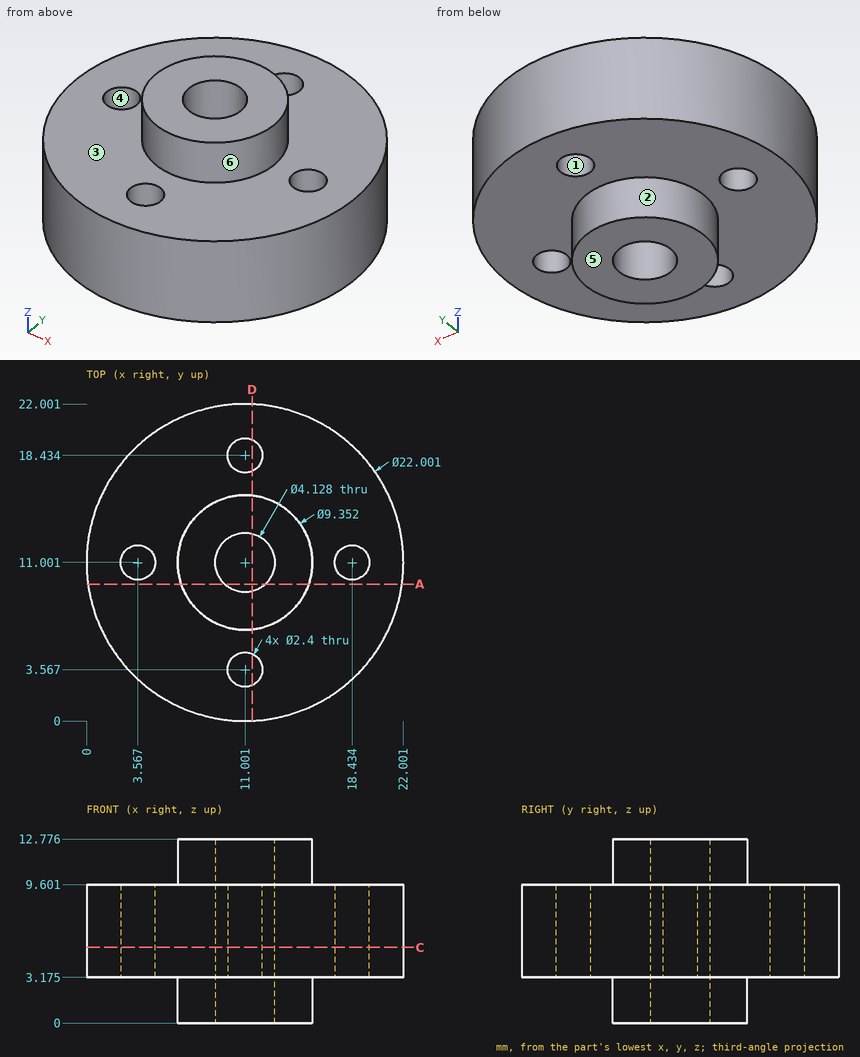
Geometry: see drawing. Coordinates: mm, zero at the bounding-box minimum. A direction names the side the tool comes from. Give positions to 0.01 mm unless a question says otherwise; leave off trailing zeros. Loops run counter-clockwise (first coordinate to the right, second up) from the corner with the lowest first, then second, coordinate; pieces in that order, holes last. Notation, with made-up numbers: (33.25, 1.25) -> (37.25, 1.25) arc R30 cw to (37.25, 31.25) -> close; hole circle Ø8 at (28.5, 7). An arc over 180 degrees is marked (long way). Use CSV: the item, a comma, the result in double quotes.
(1) Cut plane A-A (y = 9.5). Output: boundary loops of the cut face in (x, z) (1 decimal), plus the area to 3 significant figures.
From the geometry:
outline,"(0.1, 3.2) -> (6.6, 3.2) -> (6.6, 0) -> (9.6, 0) -> (9.6, 12.8) -> (6.6, 12.8) -> (6.6, 9.6) -> (0.1, 9.6) -> close; (12.4, 0) -> (15.4, 0) -> (15.4, 3.2) -> (21.9, 3.2) -> (21.9, 9.6) -> (15.4, 9.6) -> (15.4, 12.8) -> (12.4, 12.8) -> close"
area,"160 mm^2"
(2) First-contact query: P1, Ø4, axis at x = 9, y = 19.5, coming from the +Z side; P2, Ø3, axis at x = 6.5, z = 2.5, coming from the -Y side (1 decimal); P3, Ø2, axis at x = 11, y = 18.43, coming from the -Z side; P4, Ø3, axis at x = 5.5, z = 7.5, coming from the +Y side. Flat tips, straight axial feed; report the tip coordinate or a pass-through.
From the geometry:
P1,"z = 9.6"
P2,"y = 0.5"
P3,"through"
P4,"y = 21.25"
(3) Cut plane D-D (x = 11.5). Count the separate pieces of the cut face and the enclosed holes in it, plus the area to 3 significant figures.
From the geometry:
separate pieces,"4"
enclosed holes,"0"
area,"121 mm^2"
(4) Access query for the marked faces 1, 2 and 3. Directions: +Z, -Z, +X, -X, +Y, -Y. A direction counts if a zero-diameter tool reaches every point of the face in a straight line with its end or side. Return the directions, or none.
From the geometry:
face 1,"+Z, -Z"
face 2,"-Z"
face 3,"+Z"
(5) Ray query, line 1 along X through (y, z) = (11, 9.5) (1 decimal); line 2 along Z through (x, y) = (7.5, 2.5) (1 decimal); line 3 along X through (y, z) = (10.25, 11) (1 decimal). Return the intervals inside material, ascending. Write a range as [from, to].
From the geometry:
line 1,"[0, 2.4], [4.8, 8.9], [13.1, 17.2], [19.6, 22]"
line 2,"[3.2, 9.6]"
line 3,"[6.4, 9.1], [12.9, 15.6]"
(6) Cut plane C-C (z = 5.25). Output: boundary loops of the cut face in (x, y) (1 decimal).
From the geometry:
outline,"circle Ø22 at (11, 11); hole circle Ø2.4 at (3.6, 11); hole circle Ø4.1 at (11, 11); hole circle Ø2.4 at (11, 3.6); hole circle Ø2.4 at (11, 18.4); hole circle Ø2.4 at (18.4, 11)"
(7) Pull-direction query (Y, two-part tool) for the marked faces 4, 5 and 6; classes: released by +Y, released by -Y, zero draft, split by the parting line, or undercut.
From the geometry:
face 4,"undercut"
face 5,"zero draft"
face 6,"split by the parting line"
